Input: part model. Units: mm. Frame: model coordinates. A direction names the side the tool comes from. Give positions to 0.01 mm unless a question says otherwise; leave off trailing zeros. Write each loop counter-clockwise with the first axis right and the second up, starting at its lowest first coordinate (ties: lowest second). Pieces come first, ordered by that corner, then holes. Notation, with made-up numbers: (-38, 75.5) - (-30, 75.5) arc R31 cw to (-30, 108.5) - close; hole circle Ø7 at (-14.5, 47). An arc over 180 degrees is marked (long way). Use a Markdown table: item, result. Add a question column.
1. Section query D-D, the plane z = 22. Return loops of the section in (x, y).
2. Section query C-C, the plane x = -8.5. Return loops of the section in (y, z).
3. Section query B-B, the plane z = 110.5. Return loops of the section in (x, y), plus the area to 3 significant figures.
4. Mould query, pull axis Y, two halves, no side actions, for faces 3 (the flat face through (11.959, -10, 116)), 4 (the flat face through (3, 16.007, 116)), 5 (the flat face through (13.229, -9, 116)). Classes: released by +Y, released by -Y, zero draft, split by the parting line, or undercut.
5. Set-up query: faces 1 (the flat face through (-12, -9, 0)), 2 (the flat face through (-10.901, -9, 116)). Return all of +Z, -Z, +X, -X, +Y, -Y with unobstructed straight access to the full face (end or side cutting, diameter ignored); none if empty.
6. Section query A-A, the plane y = -31. Return loops of the section in (x, z).
7. Material intervals for probe 1 along X at (y, z) = (-10.5, 159); probe 2 along Y at (x, z) = (-0.5, 169.5); probe 3 along X at (y, z) = (-33.9, 190.5), sorted ascending.
Autodesk Inventor part; units mm, degrees
ref_plane "YZ Plane" through (0, 0, 0) normal (1, 0, 0) x (0, 1, 0)
ref_plane "XZ Plane" through (0, 0, 0) normal (0, 1, 0) x (-1, 0, 0)
ref_plane "XY Plane" through (0, 0, 0) normal (0, 0, 1) x (1, 0, 0)
sketch "Sketch1" plane through (0, 0, 0) normal (0, 0, 1) x (1, 0, 0)
  line L0 (-12.1708, 16.0073) -> (13.2292, 16.0073)
  line L1 (13.2292, 16.0073) -> (13.2292, -34.7927)
  line L2 (13.2292, -34.7927) -> (-12.1708, -34.7927)
  line L3 (-12.1708, -34.7927) -> (-12.1708, 16.0073)
  line L4 (11.9592, 14.7373) -> (-10.9008, 14.7373)
  line L5 (-10.9008, 14.7373) -> (-10.9008, -33.5227)
  line L6 (-10.9008, -33.5227) -> (11.9592, -33.5227)
  line L7 (11.9592, -33.5227) -> (11.9592, 14.7373)
  point P0 (0, 0)
  dimension "d0" = 25.4
  dimension "d1" = 50.8
  dimension "d2" = 1.27
extrude "Extrusion1" add sketch "Sketch1" along normal blind 234.95
sketch "Sketch2" plane through (-12.1708, 16.0073, 0) normal (0, 1, 0) x (1, 0, 0)
  circle A0 centre (12.7, -12.7) radius 1.7272
  line L0 (25.4, 0) -> (0, 0)
  line L1 (0, 0) -> (0, -234.95)
  point P0 (12.1708, 0)
  dimension "d5" = 3.4544
  dimension "d6" = 12.7
  dimension "d7" = 12.7
extrude "Extrusion2" cut sketch "Sketch2" against normal through all
pattern_linear "Rectangular Pattern1" count 23 spacing 25.4 along (0, 0, 1) of "Extrusion2"
sketch "Sketch5" plane through (13.2292, -34.7927, 0) normal (1, 0, 0) x (0, 0, -1)
  circle A0 centre (-206.375, 25.4) radius 14.2875
  line L0 (-234.95, 0) -> (-234.95, 50.8)
  line L1 (0, 50.8) -> (-234.95, 50.8)
  circle A1 centre (-28.575, 25.4) radius 14.2875
  point P0 (0, 34.7927)
  dimension "d46" = 28.575
  dimension "d47" = 28.575
  dimension "d48" = 25.4
  dimension "d52" = 28.575
  dimension "d54" = 25.4
  dimension "d61" = 28.575
extrude "Extrusion5" cut sketch "Sketch5" against normal through all
equation "\"d3\" = d13"
equation "\"d10\" = d14"
equation "\"d13\" = 234.95"
equation "\"d14\" = d13"
equation "\"d32\" = 101.6"
properties part number "AIntakeArm2"
Result sheet:
| question | item | result |
|---|---|---|
| 1 | outline | (-12.17, -34.79) - (13.23, -34.79) - (13.23, -22.08) - (11.96, -22.08) - (11.96, -33.52) - (-10.9, -33.52) - (-10.9, -22.08) - (-12.17, -22.08) - close; (-12.17, 3.29) - (-10.9, 3.29) - (-10.9, 14.74) - (11.96, 14.74) - (11.96, 3.29) - (13.23, 3.29) - (13.23, 16.01) - (-12.17, 16.01) - close |
| 2 | outline | (-34.79, 0) - (-33.52, 0) - (-33.52, 234.95) - (-34.79, 234.95) - close; (14.74, 0) - (16.01, 0) - (16.01, 234.95) - (14.74, 234.95) - close |
| 3 | outline | (-12.17, -34.79) - (13.23, -34.79) - (13.23, 16.01) - (-12.17, 16.01) - close; hole (-10.9, -33.52) - (11.96, -33.52) - (11.96, 14.74) - (-10.9, 14.74) - close |
| 3 | area | 187 mm² |
| 4 | face 3 | undercut |
| 4 | face 4 | released by +Y |
| 4 | face 5 | zero draft |
| 5 | face 1 | -Z, +X, -X, +Y, -Y |
| 5 | face 2 | +Z, -Z |
| 6 | outline | (-12.17, 0) - (-10.9, 0) - (-10.9, 234.95) - (-12.17, 234.95) - close; (11.96, 0) - (13.23, 0) - (13.23, 234.95) - (11.96, 234.95) - close |
| 7 | probe 1 | x = -12.17 to -10.9, 11.96 to 13.23 |
| 7 | probe 2 | y = -34.79 to -33.52, 14.74 to 16.01 |
| 7 | probe 3 | x = -12.17 to -1.2, 2.26 to 13.23 |
